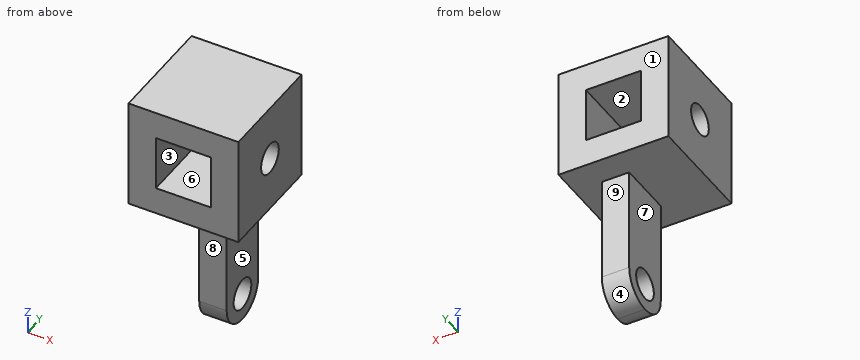
Autodesk Inventor part; units mm, degrees
ref_plane "YZ Plane" through (0, 0, 0) normal (1, 0, 0) x (0, 1, 0)
ref_plane "XZ Plane" through (0, 0, 0) normal (0, 1, 0) x (-1, 0, 0)
ref_plane "XY Plane" through (0, 0, 0) normal (0, 0, 1) x (1, 0, 0)
sketch "Sketch1" plane through (0, 0, 0) normal (0, 1, 0) x (-1, 0, 0)
  line L0 (0, 0) -> (-10, 0)
  line L1 (-10, 0) -> (-10, 10)
  line L2 (-10, 10) -> (0, 10)
  line L3 (0, 10) -> (0, 0)
  line L4 (0, 0) -> (-2.5, 0)
  line L5 (-2.5, 0) -> (-2.5, 2.5)
  line L6 (-2.5, 2.5) -> (0, 2.5)
  line L7 (0, 2.5) -> (0, 0)
  line L8 (-2.5, 2.5) -> (-7.5, 2.5)
  line L9 (-7.5, 2.5) -> (-7.5, 7.5)
  line L10 (-7.5, 7.5) -> (-2.5, 7.5)
  line L11 (-2.5, 7.5) -> (-2.5, 2.5)
  dimension "d0" = 10
  dimension "d1" = 10
  dimension "d2" = 2.5
  dimension "d3" = 2.5
  dimension "d4" = 5
  dimension "d5" = 5
extrude "Extrusion1" add sketch "Sketch1" along normal blind 10
sketch "Sketch2" plane through (10, 0, 10) normal (1, 0, 0) x (0, 0, -1)
  line L0 (10, 10) -> (0, 10)
  line L1 (0, 10) -> (5, 10)
  line L2 (5, 10) -> (5, 5)
  line L3 (5, 5) -> (0, 5)
  line L4 (0, 5) -> (0, 10)
  circle A0 centre (5, 5) radius 1.4
  point P0 (10, 0)
  dimension "d8" = 5
  dimension "d9" = 5
  dimension "d10" = 2.8
extrude "Extrusion2" cut sketch "Sketch2" against normal through all contours A0 L3 L2 | L2 L3 A0
sketch "Sketch3" plane through (10, 0, 0) normal (0, 0, -1) x (-1, 0, 0)
  line L0 (0, 10) -> (10, 10)
  line L1 (10, 10) -> (7.5, 10)
  line L2 (7.5, 10) -> (7.5, 7.5)
  line L3 (7.5, 7.5) -> (10, 7.5)
  line L4 (10, 7.5) -> (10, 10)
  line L5 (7.5, 7.5) -> (2.5, 7.5)
  line L6 (2.5, 7.5) -> (2.5, 2.5)
  line L7 (2.5, 2.5) -> (7.5, 2.5)
  line L8 (7.5, 2.5) -> (7.5, 7.5)
  line L9 (2.5, 2.5) -> (5, 2.5)
  line L10 (5, 2.5) -> (5, 7.5)
  line L11 (5, 7.5) -> (2.5, 7.5)
  line L12 (2.5, 7.5) -> (2.5, 2.5)
  point P0 (10, 0)
  dimension "d13" = 2.5
  dimension "d14" = 2.5
  dimension "d15" = 5
  dimension "d16" = 5
extrude "Extrusion3" add sketch "Sketch3" along normal blind 12 contours L10 L7 L6 L5
sketch "Sketch4" plane through (7.5, 2.5, 0) normal (1, 0, 0) x (0, 0, -1)
  line L0 (0, 5) -> (12, 5)
  line L1 (12, 5) -> (9.5, 5)
  line L2 (9.5, 5) -> (9.5, 2.5)
  line L3 (9.5, 2.5) -> (12, 2.5)
  line L4 (12, 2.5) -> (12, 5)
  circle A0 centre (9.5, 2.5) radius 1.4
  point P0 (0, -2.5)
  dimension "d19" = 2.5
  dimension "d20" = 2.5
  dimension "d21" = 2.8
extrude "Extrusion4" cut sketch "Sketch4" against normal through all contours A0 L3 L2 | L2 L3 A0
fillet "Fillet1" radius 2.5 2 edges at (6.25, 7.5, -12) (6.25, 2.5, -12)
properties part number "CAM03"
Could you check a few things on this model? Use its own coordinates, in mm. Face numbers are marked on the shaded views. A direction names the side the tool comes from. Coordinates: 2 decimals unless noted, no trailing zeros. Write each loop counter-clockwise with the first axis right and the second up, starting at its lowest first coordinate (ties: lowest second). Pieces come first, ordered by that corner, then holes. Notation, with made-up numbers: (45, 60) -> (88, 60) arc R13 cw to (88, 75) -> close; hole circle Ø10 at (-5.5, 57). An arc over 180 degrees is marked (long way). Write item = value, one per line. Start each with the question number.
(1) Which directions (+Z, -Z, +X, -X, +Y, -Y) give clear straight access to the entire face, cutting with the end or side of a thin tool? Please do the marked faces 5, 6, 7, 8 and 9.
(2) I want a section at A-A (x = 6.5). Give the number of separate pieces and of enclosed holes in the cut face, plus the area to 3 significant figures.
(3) Will these pins go through, and if not, where does the flat tip stop? pin 1 (3 mm diameter, centred on x = 6.5, z = -4, fed in from +Y); pin 2 (3 mm diameter, centred on x = 6.5, z = -3.5, fed in from -Y); pin 3 (2.5 mm diameter, centred on y = 5.5, z = -5, fed in from -X).
(4) I want a section at D-D (x = 2). Please give me the cut outline in (y, z), plus the area to 3 significant figures.
(5) I want a section at B-B (z = 5). Please give me the cut outline in (x, y), plus the area to 3 significant figures.
(6) I want a section at C-C (y = 6). Please give me the cut outline in (x, z), plus the area to 3 significant figures.
(7) I need wall thicknesses on line 1 (Z direction, x = 5.95, y = 5); line 2 (Z direction, x = 7, y = 0.5); line 3 (Z direction, x = 9.1, y = 5). Which ranges of each line are inside material? Lowest first, please. Write a range as [from, to].
(8) We'd pull the mould along Z, two halves only. Please class the marked faces 1, 2, 3 and 4: released by +Z, released by -Z, zero draft, split by the parting line, or undercut.
Result set:
q1.face_5 = -Z, +X, +Y, -Y
q1.face_6 = +Y, -Y
q1.face_7 = -Z, -X, +Y, -Y
q1.face_8 = -Z, +X, -X, -Y
q1.face_9 = -Z, +X, -X, +Y
q2.separate_pieces = 2
q2.enclosed_holes = 1
q2.area = 101 mm2
q3.pin_1 = 7.5
q3.pin_2 = 2.5
q3.pin_3 = 5
q4.outline = (0, 0) -> (10, 0) -> (10, 10) -> (0, 10) -> close; hole circle Ø2.8 at (5, 5)
q4.area = 93.8 mm2
q5.outline = (0, 0) -> (2.5, 0) -> (2.5, 3.6) -> (0, 3.6) -> close; (0, 6.4) -> (2.5, 6.4) -> (2.5, 10) -> (0, 10) -> close; (7.5, 0) -> (10, 0) -> (10, 3.6) -> (7.5, 3.6) -> close; (7.5, 6.4) -> (10, 6.4) -> (10, 10) -> (7.5, 10) -> close
q5.area = 36.0 mm2
q6.outline = (0, 0) -> (5, 0) -> (5, -8.52) -> (7.5, -8.52) -> (7.5, 0) -> (10, 0) -> (10, 4.02) -> (7.5, 4.02) -> (7.5, 2.5) -> (2.5, 2.5) -> (2.5, 4.02) -> (0, 4.02) -> close; (0, 5.98) -> (2.5, 5.98) -> (2.5, 7.5) -> (7.5, 7.5) -> (7.5, 5.98) -> (10, 5.98) -> (10, 10) -> (0, 10) -> close; (5, -11.79) -> (7.5, -11.79) -> (7.5, -10.48) -> (5, -10.48) -> close
q6.area = 89.8 mm2
q7.line_1 = [-12, -10.9], [-8.1, 2.5], [7.5, 10]
q7.line_2 = [0, 2.5], [7.5, 10]
q7.line_3 = [0, 3.6], [6.4, 10]
q8.face_1 = zero draft
q8.face_2 = undercut
q8.face_3 = undercut
q8.face_4 = released by -Z
